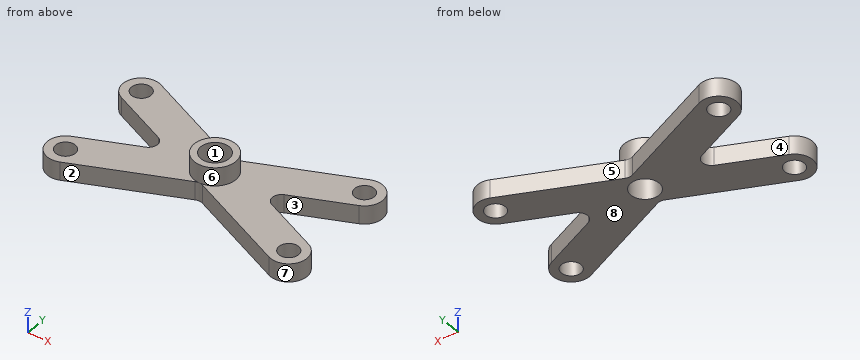
Autodesk Inventor part; units mm, degrees
ref_plane "YZ Plane" through (0, 0, 0) normal (1, 0, 0) x (0, 1, 0)
ref_plane "XZ Plane" through (0, 0, 0) normal (0, 1, 0) x (-1, 0, 0)
ref_plane "XY Plane" through (0, 0, 0) normal (0, 0, 1) x (1, 0, 0)
sketch "スケッチ1" plane through (0, 0, 0) normal (0, 0, 1) x (1, 0, 0)
  line L0 (-25, -11) -> (25, -11) construction
  line L1 (25, -11) -> (25, 11) construction
  line L2 (25, 11) -> (-25, 11) construction
  line L3 (-25, 11) -> (-25, -11) construction
  line L4 (-25, -11) -> (25, 11) construction
  line L5 (25, -11) -> (-25, 11) construction
  line L6 (25, -11) -> (-25, 11) construction
  line L7 (26.611, -7.3387) -> (-23.389, 14.6613)
  line L8 (-26.611, 7.3387) -> (23.389, -14.6613)
  arc A0 (23.389, -14.6613) -> (26.611, -7.3387) centre (25, -11) ccw
  arc A1 (-23.389, 14.6613) -> (-26.611, 7.3387) centre (-25, 11) ccw
  line L9 (-25, -11) -> (25, 11) construction
  line L10 (-23.389, -14.6613) -> (26.611, 7.3387)
  line L11 (23.389, 14.6613) -> (-26.611, -7.3387)
  arc A2 (-26.611, -7.3387) -> (-23.389, -14.6613) centre (-25, -11) ccw
  arc A3 (26.611, 7.3387) -> (23.389, 14.6613) centre (25, 11) ccw
  point P0 (0, 0)
  point P1 (0, 4.3701)
  point P2 (-9.932, 0)
  point P3 (0, -4.3701)
  point P4 (9.932, 0)
  dimension "d0" = 50
  dimension "d1" = 22
  dimension "d2" = 8
  dimension "d3" = 8
extrude "押し出し1" add sketch "スケッチ1" along normal blind 4
fillet "フィレット1" radius 2 4 edges at (0, -4.3701, 2) (-9.932, 0, 2) (0, 4.3701, 2) (9.932, 0, 2)
sketch "スケッチ2" plane through (0, 0, 4) normal (0, 0, 1) x (1, 0, 0)
  arc A0 (-23.389, 14.6613) -> (-26.611, 7.3387) centre (-25, 11) ccw
  arc A1 (-26.611, -7.3387) -> (-23.389, -14.6613) centre (-25, -11) ccw
  arc A2 (23.389, -14.6613) -> (26.611, -7.3387) centre (25, -11) ccw
  arc A3 (26.611, 7.3387) -> (23.389, 14.6613) centre (25, 11) ccw
  point P0 (0, 0)
  point P1 (-28.3993, 7.3333)
  point P2 (-28.3993, -7.3333)
  point P3 (28.3993, -7.3333)
  point P4 (28.3993, 7.3333)
hole "穴1" at (-25, 11, 4) at (25, 11, 4) at (25, -11, 4) at (-25, -11, 4) direction (0, 0, -1) diameter 4.3 end through all
sketch "スケッチ3" plane through (0, 0, 4) normal (0, 0, 1) x (1, 0, 0)
  circle A0 centre (0, 0) radius 3.1
  dimension "d15" = 6.2
extrude "押し出し2" cut sketch "スケッチ3" against normal blind 8
sketch "スケッチ4" plane through (0, 0, 4) normal (0, 0, 1) x (1, 0, 0)
  circle A0 centre (0, 0) radius 3.1
  circle A1 centre (0, 0) radius 4.5551
  arc A2 (-0.8055, 4.7245) -> (0.8055, 4.7245) centre (0, 6.5551) ccw
extrude "押し出し3" add sketch "スケッチ4" along normal blind 4
properties part number "base21" material "ABS プラスチック"
Can you work these out from the model? Positions are in its coordinate system, mm. Face numbers are marked on the shaded views. A direction names the side the tool comes from. Give positions to 0.01 mm unless a question says otherwise; leave off trailing zeros. Order: outer loops, then holes, each group sorted by start corner. A loop starts at its lowest first (then second) coordinate and runs counter-clockwise, first axis right, second up. Notation, with made-up numbers: M 70.25,-35.5 L 101.25,-35.5 A18 ccw 101.25,-15.5 Z; hole C 57.5,12 d7. An arc over 180 degrees is marked long. One line per item, written item: value.
Item 1: If we mould it in two halves opening along Y, with no side actions, what happens to the marked faces 6, 7 and 8? For each: pulls with the +Y half, pulls with the -Y half, needs draft (parallel to the pull), parting line crosses it, or undercut.
Verdict:
face 6: parting line crosses it
face 7: undercut
face 8: needs draft
Item 2: For the marked faces 1, 2, 3, 4 and 5, which set-ups out of +Z, -Z, +X, -X, +Y, -Y let a thin tool reach every point of the face, with its end or its side?
Verdict:
face 1: +Z, -Z
face 2: +Z, -Z, -Y
face 3: +Z, -Z, +X
face 4: +Z, -Z, -X
face 5: +Z, -Z, +Y
Item 3: If we section it at D-D on y = -12: Write out the boundary of the cut face in (x, z).
Verdict:
outline: M -28.87,0 L -26.9,0 L -26.9,4 L -28.87,4 Z; M -23.1,0 L -17.34,0 L -17.34,4 L -23.1,4 Z; M 17.34,0 L 23.1,0 L 23.1,4 L 17.34,4 Z; M 26.9,0 L 28.87,0 L 28.87,4 L 26.9,4 Z
Item 4: Please list where these lines run through material, in increasing order: line 1 (Y direction, x = 0, z = 0.5); line 2 (Y direction, x = -25, z = 2.3); line 3 (X direction, y = -11, z = 2.65).
Verdict:
line 1: -4.56 to -3.1, 3.1 to 4.56
line 2: -15 to -13.15, -8.85 to -6.63, 6.63 to 8.85, 13.15 to 15
line 3: -29 to -27.15, -22.85 to -15.07, 15.07 to 22.85, 27.15 to 29
Item 5: If we section it at A-A on y = 0: Write out the boundary of the cut face in (x, z), and give its area (3 significant figures).
Verdict:
outline: M -12.9,0 L -3.1,0 L -3.1,8 L -4.56,8 L -4.56,4 L -12.9,4 Z; M 3.1,0 L 12.9,0 L 12.9,4 L 4.56,4 L 4.56,8 L 3.1,8 Z
area: 90.0 mm2
Item 6: For pin 1 (4 mm diameter, centred on y = 7.5, z = 5.5, fed in from +X); pin 2 (2.5 mm diameter, centred on x = -25, y = 11, fed in from +Z); pin 3 (5.5 mm diameter, centred on x = 25, y = 11, fed in from -Z); pin 4 (12 mm diameter, centred on x = -13.5, y = -11.5, fed in from +Z), each with a flat end and sliding along its axis, tell me the tip position at first contact or that it passes through.
Verdict:
pin 1: x = 28.36
pin 2: through
pin 3: z = 0
pin 4: z = 4
Item 7: If we section it at C-C on x = 17: Write out the boundary of the cut face in (y, z), and give its area (3 significant figures).
Verdict:
outline: M -11.85,0 L -3.11,0 L -3.11,4 L -11.85,4 Z; M 3.11,0 L 11.85,0 L 11.85,4 L 3.11,4 Z
area: 69.9 mm2
Item 8: If we section it at B-B on z = 2.5: Write out the boundary of the cut face in (x, y).
Verdict:
outline: M -26.61,-7.34 A4 ccw -23.39,-14.66 L -0.81,-4.72 A2 cw 0.81,-4.72 L 23.39,-14.66 A4 ccw 26.61,-7.34 L 14.09,-1.83 A2 cw 14.09,1.83 L 26.61,7.34 A4 ccw 23.39,14.66 L 0.81,4.72 A2 cw -0.81,4.72 L -23.39,14.66 A4 ccw -26.61,7.34 L -14.09,1.83 A2 cw -14.09,-1.83 Z; hole C -25,-11 d4.3; hole C -25,11 d4.3; hole C 0,0 d6.2; hole C 25,-11 d4.3; hole C 25,11 d4.3
